from build123d import *

# Parameters (mm, degrees)
SKETCH1_W                      = 140
SKETCH1_H                      = 160
BOSS_EXTRUDE1_DEPTH            = 7
CBORE_FOR_M4_SHCS1_D           = 4.8
CBORE_FOR_M4_SHCS1_CBORE_D     = 8
CBORE_FOR_M4_SHCS1_CBORE_DEPTH = 4
CHAMFER1_SIZE                  = 10
CUT_EXTRUDE1_REACH             = 108.532
SKETCH8_W                      = 85
SKETCH8_H                      = 120
FILLET1_R                      = 10
SKETCH9_W                      = 85
SKETCH9_H                      = 20
BOSS_EXTRUDE3_DEPTH            = 7
FILLET2_R                      = 10
M3_CLEARANCE_HOLE1_OUTLINE_R   = 1.8
M3_CLEARANCE_HOLE1_DEPTH       = 7


# Read off the part's stored shape, not the designer's step: M3 Clearance Hole1
with BuildPart() as part:
    # Sketch1 → Boss-Extrude1 (new body)
    with BuildSketch(Plane(origin=(0, 0, 0), x_dir=(1, 0, 0), z_dir=(0, 1, 0))):
        Rectangle(SKETCH1_W, SKETCH1_H)
    extrude(amount=BOSS_EXTRUDE1_DEPTH)

    # CBORE for M4 SHCS1 (through all)
    with Locations(Plane(origin=(0, 7, 0), x_dir=(1, 0, 0), z_dir=(0, 1, 0))):
        with Locations((-56, 38), (56, 38), (-56, -7), (56, 0), (-56, -52), (56, -52)):
            CounterBoreHole(CBORE_FOR_M4_SHCS1_D / 2, CBORE_FOR_M4_SHCS1_CBORE_D / 2, CBORE_FOR_M4_SHCS1_CBORE_DEPTH)

    # Chamfer1
    chamfer1_edges = [part.edges().sort_by_distance(p)[0] for p in [
        (70, 3.5, 80),
        (-70, 3.5, 80),
        (-70, 3.5, -80),
        (70, 3.5, -80),
    ]]
    chamfer(chamfer1_edges, length=CHAMFER1_SIZE)

    # Sketch8 → Cut-Extrude1 (cut, up to next)
    with BuildSketch(Plane.XZ, mode=Mode.PRIVATE) as cut_extrude1_sk1:
        Rectangle(SKETCH8_W, SKETCH8_H)
    cut_extrude1_tool1 = extrude(cut_extrude1_sk1.sketch, amount=-CUT_EXTRUDE1_REACH, mode=Mode.PRIVATE) & part.part
    add(cut_extrude1_tool1.solids().sort_by_distance((0, 0, 0))[0], mode=Mode.SUBTRACT)

    # Fillet1
    fillet1_edges = [part.edges().sort_by_distance(p)[0] for p in [
        (-42.5, 3.5, -60),
        (-42.5, 3.5, 60),
        (42.5, 3.5, 60),
        (42.5, 3.5, -60),
    ]]
    fillet(fillet1_edges, radius=FILLET1_R)

    # Sketch9 → Boss-Extrude3 (add)
    with BuildSketch(Plane.XZ):
        Rectangle(SKETCH9_W, SKETCH9_H)
    extrude(amount=-BOSS_EXTRUDE3_DEPTH)

    # Fillet2
    fillet2_edges = [part.edges().sort_by_distance(p)[0] for p in [
        (42.5, 3.5, 10),
        (42.5, 3.5, -10),
        (-42.5, 3.5, -10),
        (-42.5, 3.5, 10),
    ]]
    fillet(fillet2_edges, radius=FILLET2_R)

    # M3 Clearance Hole1 outline → M3 Clearance Hole1 (cut)
    with BuildSketch(Plane(origin=(0, 0, 0), x_dir=(1, 0, 0), z_dir=(0, 1, 0))):
        with Locations((60, -70)):
            Circle(M3_CLEARANCE_HOLE1_OUTLINE_R)
        with Locations((-60, 70)):
            Circle(M3_CLEARANCE_HOLE1_OUTLINE_R)
        with Locations((-60, -70)):
            Circle(M3_CLEARANCE_HOLE1_OUTLINE_R)
        with Locations((60, 70)):
            Circle(M3_CLEARANCE_HOLE1_OUTLINE_R)
        Circle(M3_CLEARANCE_HOLE1_OUTLINE_R)
    extrude(amount=M3_CLEARANCE_HOLE1_DEPTH, mode=Mode.SUBTRACT)


solid = part.part
Work out the finished part from the listing and answer in its coordinate system (mm). A direction names the side the tool comes from. Give positions to 0.01 mm unless a question says otherwise; leave off trailing zeros. Order: outer loops, then holes, each group sorted by start corner. A loop starts at its lowest first (then second) coordinate and runs counter-clockwise, first axis right, second up. Notation, with made-up numbers: M -15,-30 L 30,-30 A34 ccw 30,2 Z; hole C 56.25,-40 d3. An arc over 180 degrees is marked long. Return JSON: item names as keys, results as strings.
Q1. Find section B-B, the plane x = 56. Write down the section's boundary in (y, z).
Answer below:
{"outline": "M 0,-80 L 7,-80 L 7,-42 L 3,-42 L 3,-40.4 L 0,-40.4 Z; M 0,-35.6 L 3,-35.6 L 3,-34 L 7,-34 L 7,-4 L 3,-4 L 3,-2.4 L 0,-2.4 Z; M 0,2.4 L 3,2.4 L 3,4 L 7,4 L 7,48 L 3,48 L 3,49.6 L 0,49.6 Z; M 0,54.4 L 3,54.4 L 3,56 L 7,56 L 7,80 L 0,80 Z"}
Q2. Find section A-A, the plane z = 27.5. Write down the section's boundary in (x, y).
Answer below:
{"outline": "M -70,0 L -42.5,0 L -42.5,7 L -70,7 Z; M 42.5,0 L 70,0 L 70,7 L 42.5,7 Z"}
Q3. Find section D-D, the plane z = -38. Write down the section's boundary in (x, y), and give its area (3 significant figures).
Answer below:
{"outline": "M -70,0 L -58.4,0 L -58.4,3 L -60,3 L -60,7 L -70,7 Z; M -53.6,0 L -42.5,0 L -42.5,7 L -52,7 L -52,3 L -53.6,3 Z; M 42.5,0 L 53.6,0 L 53.6,3 L 52,3 L 52,7 L 42.5,7 Z; M 58.4,0 L 70,0 L 70,7 L 60,7 L 60,3 L 58.4,3 Z", "area": "292 mm^2"}
Q4. Find the intervals of material crossed by line 1 along Z through (x, y) = (19.5, 1); line 2 along X through (y, z) = (0.5, 40.5); line 3 along X through (y, z) = (1.5, -70), in increasing order. Write a range as [from, to].
Answer below:
{"line 1": "z = [-80, -60], [-10, 10], [60, 80]", "line 2": "x = [-70, -42.5], [42.5, 70]", "line 3": "x = [-70, -61.8], [-58.2, 58.2], [61.8, 70]"}
Q5. This flat-tipped pin is pushed along its axis until it touches: pin 1 (6.5 mm diameter, centred on x = 56.5, z = 52, fed in from +Y). Where does it stop, or does it pass through?
Answer below:
{"pin 1": "stops at y = 3"}
Q6. Find section C-C, the plane x = 15. Write down the section's boundary in (y, z).
Answer below:
{"outline": "M 0,-80 L 7,-80 L 7,-60 L 0,-60 Z; M 0,-10 L 7,-10 L 7,10 L 0,10 Z; M 0,60 L 7,60 L 7,80 L 0,80 Z"}
Q7. The mould has two halves that part along Z. Classify faces 1 (the face through (54.89, 1.48, 54.13)), 2 (the face through (-65, 3, -75)), 3 (the face through (-1, 3, 80)): pulls with the +Z half, pulls with the -Z half, needs draft (parallel to the pull), parting line crosses it, or undercut.
Answer below:
{"face 1": "undercut", "face 2": "pulls with the -Z half", "face 3": "pulls with the +Z half"}
Q8. Which of the six approach directions +Z, -Z, +X, -X, +Y, -Y give full straight-line access (tool end or side, diameter ignored) to faces 4 (the face through (-1, 3, -80)), 5 (the face through (59.815, 5.028, -1.201)), 6 (the face through (39.65, 3.55, -13.01))?
Answer below:
{"face 4": "-Z, +X, -X, +Y, -Y", "face 5": "+Y", "face 6": "+Y, -Y"}
